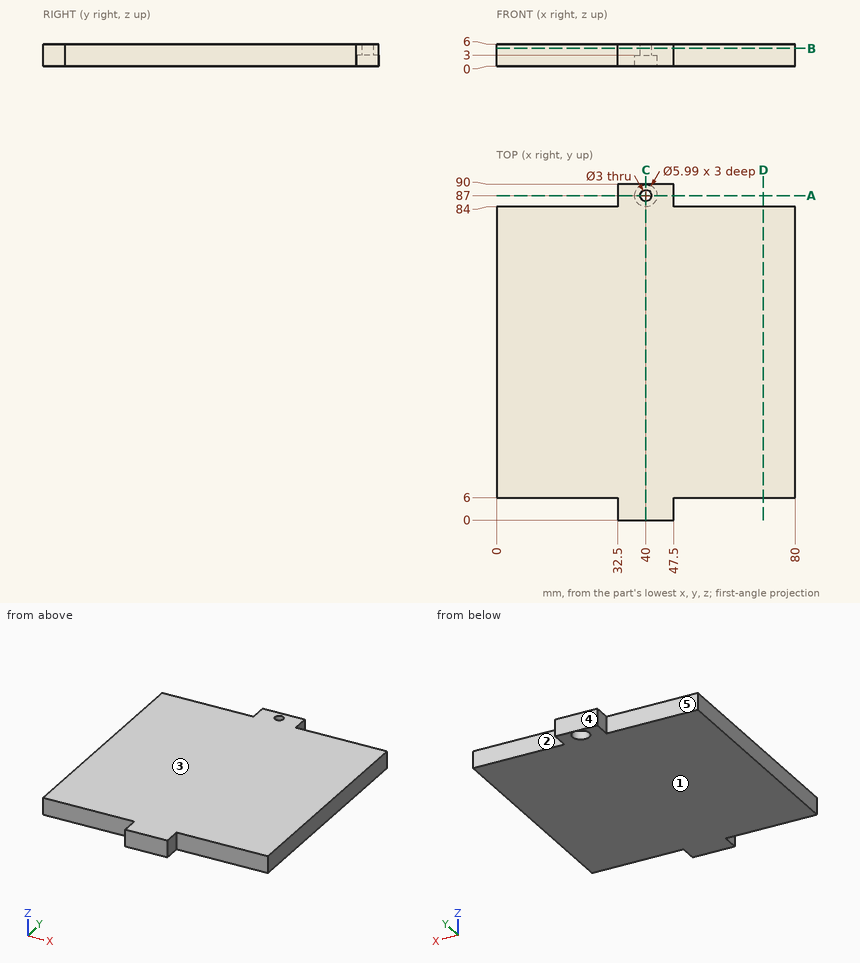
Drawing for the job (mm, zero at the part's lowest x, y, z). A direction names the side the tool comes from. Give positions to 0.01 mm unless a question says otherwise; leave off trailing zeros. Order: outer loops, then holes, each group sorted by start corner. A loop starts at its lowest first (then second) coordinate and runs counter-clockwise, first axis right, second up. Notation, with made-up numbers: M 0,-7.5 L 43,-7.5 A7 ccw 43,-1.5 Z; hole C 50.5,77 d3. An arc over 180 degrees is marked long. Use a Markdown table: item, result. Add a question column.
(1) Saw through at C-C, the plane x = 40. Give the cut face in (y, z) (3 decimals), and give its area (3 significant figures).
(2) Drop flat-ended pins along their axis: P1, Ø3, axis at x = 18.5, z = 2.5, coming from the -Y side; P2, Ø1, axis at x = 10, z = 1.5, coming from the +Y side; P3, Ø1.8, axis at y = 4, z = 3, coming from the -X side. Give the stop position or say it passes through.
(3) Saw through at D-D, the plane x = 71.5. Give the cut face in (y, z).
(4) Saw through at B-B, the plane z = 4.8. Give the cut face in (x, y), and give its area (3 significant figures).
(5) Probe line 1 along X through (y, z) = (87, 5); line 2 along Y through (x, z) = (40, 5.2); line 3 along X through (y, z) = (4, 1.05). List the from-to ranges inside material, lowest first. Write a range as [from, to].
(6) Mould opens along Z. For the marked faces 1, 2 and 3 say: +Z half, -Z half, draft (parallel to the pull), parting line (faces both ways), or undercut.
(7) 3-axis set-ups, long thin cutter, end or side, ignore diameter. For the marked faces 4 and 5: which of +Z, -Z, +X, -X, +Y, -Y reach the whole face in a straight line?
(8) Saw through at A-A, the plane y = 87. Give the cut face in (x, z) (3 decimals), and give its area (3 significant figures).
Answer key:
| question | item | result |
|---|---|---|
| 1 | outline | M 0,0 L 84.005,0 L 84.005,3 L 85.5,3 L 85.5,6 L 0,6 Z; M 88.5,3 L 89.995,3 L 89.995,0 L 90,0 L 90,6 L 88.5,6 Z |
| 1 | area | 513 mm^2 |
| 2 | P1 | y = 6 |
| 2 | P2 | y = 84 |
| 2 | P3 | x = 32.5 |
| 3 | outline | M 6,0 L 84,0 L 84,6 L 6,6 Z |
| 4 | outline | M 0,6 L 32.5,6 L 32.5,0 L 47.5,0 L 47.5,6 L 80,6 L 80,84 L 47.5,84 L 47.5,90 L 32.5,90 L 32.5,84 L 0,84 Z; hole C 40,87 d3 |
| 4 | area | 6,410 mm^2 |
| 5 | line 1 | [32.5, 38.5], [41.5, 47.5] |
| 5 | line 2 | [0, 85.5], [88.5, 90] |
| 5 | line 3 | [32.5, 47.5] |
| 6 | face 1 | -Z half |
| 6 | face 2 | draft |
| 6 | face 3 | +Z half |
| 7 | face 4 | +Z, -Z, +X, -X, +Y |
| 7 | face 5 | +Z, -Z, -X, +Y |
| 8 | outline | M 32.5,0 L 37.005,0 L 37.005,3 L 38.5,3 L 38.5,6 L 32.5,6 Z; M 41.5,3 L 42.995,3 L 42.995,0 L 47.5,0 L 47.5,6 L 41.5,6 Z |
| 8 | area | 63.0 mm^2 |
